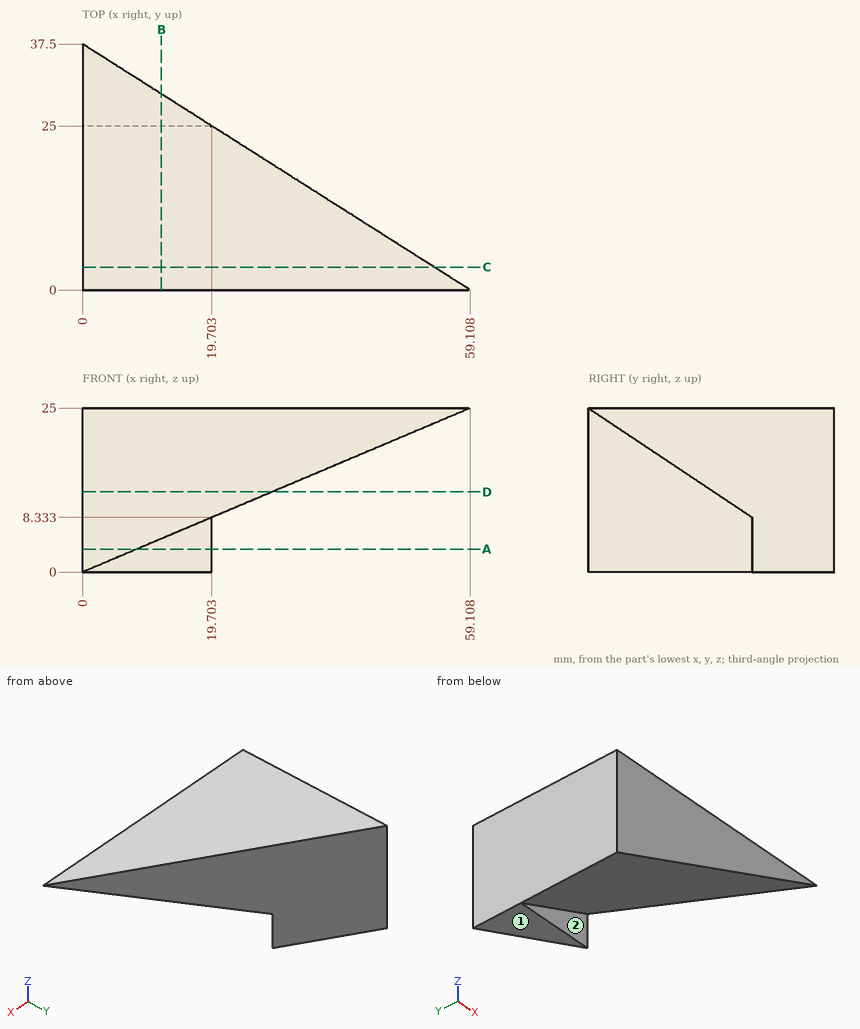
Verification items for this drawing (mm, ordinates from the low corner). A direction names the side the tool comes from. Coordinates: 2 decimals unless noted, no trailing zeros. Write each loop counter-clockwise with the first axis right and the second up, starting at its lowest first coordinate (ties: lowest second). Pieces come first, ordered by that corner, then holes. Notation, with made-up numbers: M -34,34 L -22,34 A26 cw -22,73 Z; hole C 51.25,-33.5 d11. An arc over 180 degrees is marked long. Use one line per item in the form item = value. Start each with the question number.
1) Go/stop test with flat-tipped pins: pin 1 Ø6 at (x, z) = (22.5, 3.5) entering from -Y; pin 2 Ø8 at (x, y) = (15.5, 31) entering from +Z; pin 3 Ø5 at (y, z) = (16.5, 20.5) entering from +X; pin 4 Ø3 at (y, z) = (27.5, 8.5) entering from +X (1 decimal). Record where each tip stops, or that it passes through.
2) Section check C-C on y = 3.5. Enter the section's corners in (x, z).
3) Section check B-B on x = 12. Enter the section's corners in (y, z) (1 decimal), and give its area (3 significant figures).
4) Set-up check for the marked faces 1 and 2: record each of +Z, -Z, +X, -X, +Y, -Y from which the full face is reachable in a straight line by a thin tool's end or side.
5) Section check D-D on z = 12.25. Enter the section's corners in (x, y) (1 decimal), and give its area (3 significant figures).
6) Section check A-A on z = 3.5. Enter the section's corners in (x, y) (1 decimal), and give its area (3 significant figures).
7) Thickness scan on probe 1 along X at (y, z) = (21.5, 2.75) (1 decimal); probe 2 along Z at (x, y) = (39, 3) (1 decimal); probe 3 along Y at (x, z) = (14, 4.25). Record the ranges inside material, lowest first. Write a range as from..to.
Responses:
q1.pin_1 = 25
q1.pin_2 = 25
q1.pin_3 = 37.04
q1.pin_4 = 18.1
q2.outline = M 0,0 L 53.59,22.67 L 53.59,25 L 0,25 Z
q3.outline = M 0,5.1 L 25,5.1 L 25,0 L 29.9,0 L 29.9,25 L 0,25 Z
q3.area = 620 mm2
q4.face_1 = -Z, +X, -X, +Y, -Y
q4.face_2 = -Z, +X, -Y
q5.outline = M 0,0 L 29,0 L 29,19.1 L 0,37.5 Z
q5.area = 820 mm2
q6.outline = M 0,0 L 8.3,0 L 8.3,25 L 19.7,25 L 0,37.5 Z
q6.area = 330 mm2
q7.probe_1 = 0..6.5
q7.probe_2 = 16.5..25
q7.probe_3 = 25..28.62
